Here's the drawing with two shaded views (mm, measured from the low corner). I have some questions. Round coordinates to 2 decimals unless told otherwise and drop trailing zeros. Loops run counter-clockwise (first coordinate to the right, second up) from the corner with the lowest first, then second, coordinate; pieces in that order, holes last.
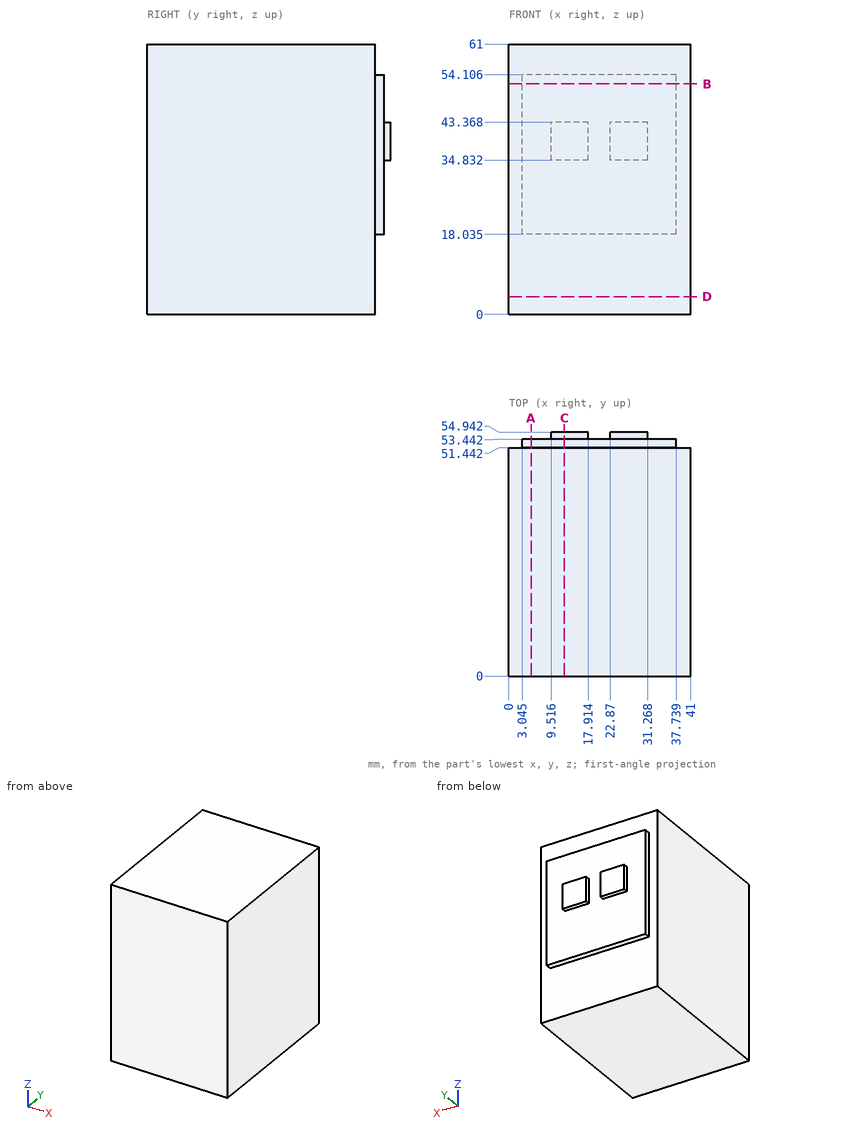
Item 1: If we section it at A-A, the plane x = 5: Please give me the cut outline in (y, z) (1 decimal), then the cut area to 3 significant figures.
Results list:
outline: (0, 0) - (51.4, 0) - (51.4, 18) - (53.4, 18) - (53.4, 54.1) - (51.4, 54.1) - (51.4, 61) - (0, 61) - close
area: 3,210 mm2
Item 2: If we section it at D-D, the plane z = 4: Please give me the cut outline in (x, y).
Results list:
outline: (0, 0) - (41, 0) - (41, 51.44) - (0, 51.44) - close
Item 3: If I drill on line 1 along Y through (x, z) = (12, 33); line 2 along Y through (x, z) = (30, 13.5); line 3 along X through (y, z) = (52.5, 25) (1 decimal), over which ranges is the centre line in solid material (lowest first)?
Results list:
line 1: y = 0 to 53.44
line 2: y = 0 to 51.44
line 3: x = 3 to 37.7
Item 4: Will these pins go through, and if not, where does the flat tip stop? pin 1 (1.6 mm diameter, centred on y = 54, z = 40.5, fed in from +X); pin 2 (0.8 mm diameter, centred on x = 12, y = 54, fed in from +Z); pin 3 (1.6 mm diameter, centred on x = 26, y = 54, fed in from -Z) (1 decimal).
Results list:
pin 1: stops at x = 37.74
pin 2: stops at z = 43.37
pin 3: stops at z = 18
Item 5: If we section it at C-C, the plane x = 12.5: Please give me the cut outline in (y, z) (1 decimal), then the cut area to 3 significant figures.
Results list:
outline: (0, 0) - (51.4, 0) - (51.4, 18) - (53.4, 18) - (53.4, 34.8) - (54.9, 34.8) - (54.9, 43.4) - (53.4, 43.4) - (53.4, 54.1) - (51.4, 54.1) - (51.4, 61) - (0, 61) - close
area: 3,220 mm2
Item 6: If we section it at B-B, the plane z = 52: Please give me the cut outline in (x, y) (1 decimal), then the cut area to 3 significant figures.
Results list:
outline: (0, 0) - (41, 0) - (41, 51.4) - (37.7, 51.4) - (37.7, 53.4) - (3, 53.4) - (3, 51.4) - (0, 51.4) - close
area: 2,180 mm2
